Verification items for the finished model (mm, model axes). A direction names the side the tool comes from. Give positions to 0.01 mm unless a question says otherwise; leave off trailing zeros. Order: outer loops, then holes, each group sorted by start corner. A loop starts at its lowest first (then second) coordinate and runs counter-clockwise, first axis right, second up. Notation, with made-up numbers: (-1.5, 1) - (18.5, 1) arc R15 cw to (18.5, 8) - close; hole circle Ø10 at (-32.5, 42.5). An arc over 180 degrees is marked (long way). Answer as a JSON object with one key per item and string values. Group by question number.
(1) Section check A-A (x = -1.5). Record the boundary of the cut face in (y, z) (3 decimals).
(2) Thickness scan on line 1 (X direction, y = 14, z = 0) (3 decimals); line 2 (X direction, y = 21, z = -19.5); line 3 (Y direction, x = 3.5, z = 4) (3 decimals). Record the ranges inside material, lowest first.
(3) Access from +Z, -Z, +X, -X, +Y, -Y to the whole of each face (thin tool, end or side, straight path). Record for faces 1 (the face through (2.54, 25, -24)), 2 (the face through (0.17, 12.7, 19.92)), 3 (the face through (0, 12.7, -25.2)), 4 (the face through (-2.54, 25, -24)), 5 (the face through (-5.54, 38.99, 19.92)).
(4) Section check D-D (x = -12.5). Record the boundary of the cut face in (y, z) (3 decimals), then the cut area to 3 significant figures.
(5) Mould release check, pull along X, two halves, no side actions. Record for faces 6 (the face through (0, 3.175, 0)), 7 (the face through (-3.83, 25.04, -30.5)), 8 (the face through (0, 25, -31.75)): +X half, -X half, draft (parallel to the pull), parting line (faces both ways), or undercut.
(6) Depth check by flat-ended pin: pin 1 Ø1.5 at (x, y) = (-14.5, 17.5) entering from +Z; pin 2 Ø10 at (y, z) = (21, -12) entering from -X; pin 3 Ø2 at (x, y) = (-14, 19.5) entering from -Z; pin 4 Ø3.5 at (y, z) = (14.99, -25.29) entering from -X. Enter the tip coordinate at first touch or a pass-through.
(7) Section check C-C (z = 3.5). Record the boundary of the cut face in (x, y) (3 decimals), then the cut area to 3 significant figures.
Autodesk Inventor part; units mm, degrees
ref_plane "YZ Plane" through (0, 0, 0) normal (1, 0, 0) x (0, 1, 0)
ref_plane "XZ Plane" through (0, 0, 0) normal (0, 1, 0) x (-1, 0, 0)
ref_plane "XY Plane" through (0, 0, 0) normal (0, 0, 1) x (1, 0, 0)
sketch "Sketch1" plane through (0, 0, 0) normal (0, 1, 0) x (-1, 0, 0)
  line L0 (0, 0) -> (0, 28.1143)
  line L1 (16.7843, 9.0105) -> (8.6989, 21.4436)
  line L2 (-8.6989, 21.4436) -> (-15.9171, 10.4666)
  arc A0 (-15.9171, 10.4666) -> (15.0435, 11.6875) centre (0, 0) ccw
  arc A1 (8.6989, 21.4436) -> (-8.6989, 21.4436) centre (0, 15.7866) ccw
extrude "Extrusion1" add sketch "Sketch1" along normal blind 50.8 contours A0 L2 A1 L1
sketch "Sketch2" plane through (0, 50.8, 0) normal (0, 1, 0) x (1, 0, 0)
  circle A0 centre (0, 0) radius 15.875
  dimension "d3" = 31.75
extrude "Extrusion2" cut sketch "Sketch2" against normal blind 47.625
sketch "Sketch3" plane through (0, 0, 0) normal (0, 0, 1) x (1, 0, 0)
  line L0 (0, 0) -> (0, 12.7)
  line L1 (-7.7476, 33.5742) -> (-7.7472, 20.4468)
  line L2 (7.7474, 33.5741) -> (7.7474, 33.574)
  line L3 (7.747, 25.8264) -> (7.7468, 20.4467)
  line L4 (7.7473, 41.3219) -> (-0.0002, 41.3219)
  arc A0 (0, 41.3219) -> (-7.7476, 33.5742) centre (-0.0001, 33.5744) ccw
  arc A1 (-7.7472, 20.4468) -> (7.7468, 20.4467) centre (-0.0002, 20.447) ccw
  arc A2 (7.747, 25.8264) -> (7.7473, 41.3219) centre (7.7474, 33.5741) ccw
  dimension "d6" = 12.7
extrude "Extrusion3" cut sketch "Sketch3" along normal blind 44.45
sketch "Sketch4" plane through (0, 0, 0) normal (1, 0, 0) x (0, 1, 0)
  arc A0 (25.8264, -0.0001) -> (41.32, -0.0702) centre (33.573, -0.0696) ccw
  line L0 (41.32, -0.0702) -> (41.32, 29.3277)
  line L1 (41.32, 29.3277) -> (25.8264, 29.047)
  line L2 (25.8264, 29.047) -> (25.8264, -0.0001)
  point P0 (0, 0)
  point P1 (25.8264, 17.4036)
extrude "Extrusion4" cut sketch "Sketch4" along normal blind 44.45
sketch "Sketch5" plane through (0, 0, 0) normal (0, -1, 0) x (1, 0, 0)
  arc A0 (-16.7843, 9.0105) -> (15.9171, 10.4666) centre (0, 0) ccw
  line L0 (0, -19.05) -> (0, -31.75)
  line L1 (2.54, -18.8799) -> (2.54, -29.21)
  line L2 (-2.54, -18.8799) -> (-2.54, -29.21)
  line L3 (5.08, -31.75) -> (2.54, -29.21)
  line L4 (-5.08, -31.75) -> (-2.54, -29.21)
  line L5 (5.08, -31.75) -> (-5.08, -31.75)
  arc A1 (-2.54, -18.8799) -> (2.54, -18.8799) centre (0, 0.0817) ccw
  dimension "d13" = 12.7
  dimension "d14" = 5.08
  dimension "d27" = 10.16
extrude "Extrusion5" add sketch "Sketch5" against normal blind 50.8
sketch "Sketch6" plane through (0, 0, 0) normal (1, 0, 0) x (0, 1, 0)
  line L0 (0, -31.75) -> (50.8, -31.75)
  circle A0 centre (35.814, -25.2921) radius 2.286
  circle A1 centre (14.986, -25.2921) radius 2.286
  line L1 (0, -25.2921) -> (12.7, -25.2921)
  line L2 (38.1, -25.2921) -> (50.8, -25.2921)
  line L3 (50.8, -19.05) -> (50.8, 10.4666)
  point P0 (0, 0)
  point P1 (50.8, 9.0105)
  dimension "d19" = 4.572
  dimension "d20" = 4.572
  dimension "d23" = 12.7
  dimension "d24" = 12.7
extrude "Extrusion6" cut sketch "Sketch6" along normal mid plane 44.45
properties part number "bikeLockMountV2part1"
Solutions:
{
 "1": {"outline": "(0, -31.75) - (50.8, -31.75) - (50.8, -15.804) - (3.175, -15.804) - (3.175, 15.804) - (12.847, 15.804) - (12.847, 26.054) - (0, 26.054) - close; (41.175, 15.804) - (50.8, 15.804) - (50.8, 26.054) - (41.175, 26.054) - close; hole circle Ø4.572 at (14.986, -25.292); hole circle Ø4.572 at (35.814, -25.292)"},
 "2": {"line 1": "x = -19.05 to -15.875, 15.875 to 19.05", "line 2": "x = -2.54 to 2.54", "line 3": "y = 0 to 3.175"},
 "3": {"face 1": "+X, +Y, -Y", "face 2": "+Z", "face 3": "+X, -X", "face 4": "-X, +Y, -Y", "face 5": "+Z, +X"},
 "4": {"outline": "(0, -14.375) - (50.8, -14.375) - (50.8, -9.786) - (3.175, -9.786) - (3.175, 9.786) - (50.8, 9.786) - (50.8, 15.599) - (0, 15.599) - close", "area": "591 mm2"},
 "5": {"face 6": "undercut", "face 7": "-X half", "face 8": "draft"},
 "6": {"pin 1": "stops at z = 13.68", "pin 2": "stops at x = -17.72", "pin 3": "stops at z = -13.92", "pin 4": "passes through"},
 "7": {"outline": "(-18.726, 0) - (18.726, 0) - (18.726, 25.826) - (15.484, 25.826) - (15.484, 3.175) - (-15.484, 3.175) - (-15.484, 50.8) - (-18.726, 50.8) - close; (15.484, 41.32) - (18.726, 41.32) - (18.726, 50.8) - (15.484, 50.8) - close", "area": "377 mm2"}
}
